Here's how the part is built. I have some questions about the finished solid (model axes, mm). Coordinates: 2 decimals unless noted, no trailing zeros. Order: outer loops, then holes, each group sorted by start corner. A loop starts at its lowest first (then second) coordinate and runs counter-clockwise, first axis right, second up. Notation, with made-up numbers: (-29, -17) - (26, -17) arc R17 ccw to (26, 1) - close; hole circle Ø1 at (75, -1). An arc over 180 degrees is marked (long way). Answer as CSV lines item,"result". Start each with the question number.
Item 1: Imagine slicing it at A-A on y = 30.5. List the corners of the cut face in (x, z) for me (3 decimals).
Item 2: Imagine slicing it at B-B on z = 250. List the corners of the cut face in (x, y) for me (3 decimals).
Item 3: I'm going to push flat-ended pins straight in: pin 1 (2.5 mm diameter, centred on x = 0, z = 241.3, fed in from +Y) (3 decimals); pin 2 (5 mm diameter, centred on x = 0, z = 139.7, fed in from +Y); pin 3 (12 mm diameter, centred on x = -2.5, y = -26, fed in from +Z). Where does each tip first touch, or does it pass through?
Item 4: I need wall thicknesses on line 1 (Y direction, x = 3.25, z = 158) (3 decimals); line 2 (X direction, y = 37.3, z = 165.1); line 3 (X direction, y = -7, z = 205) (3 decimals). Which ranges of each line are inside material? Lowest first, please.
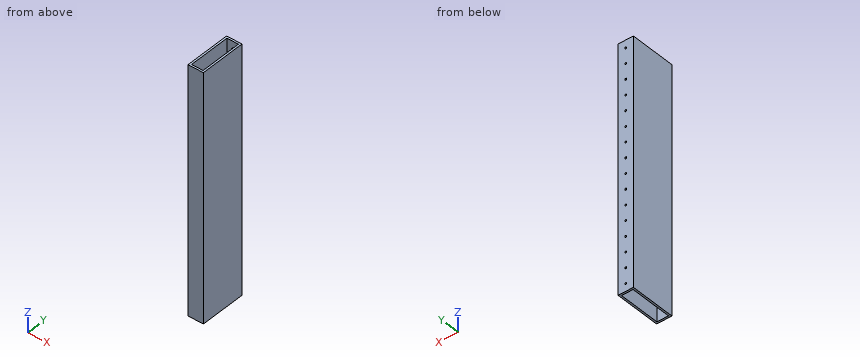
from build123d import *

# Parameters (mm, degrees)
SKETCH1_W           = 25.4
SKETCH1_H           = 76.2
BOSS_EXTRUDE1_DEPTH = 406.4
SHELL1_T            = -3.175
SKETCH2_R           = 1.5875
CUT_EXTRUDE1_DEPTH  = 3.175
LPATTERN1_COUNT     = 16
LPATTERN1_PITCH     = 25.4


with BuildPart() as part:
    # Sketch1 → Boss-Extrude1 (new body)
    with BuildSketch(Plane.XY):
        Rectangle(SKETCH1_W, SKETCH1_H)
    extrude(amount=BOSS_EXTRUDE1_DEPTH)

    # Shell1
    shell1_openings = [part.faces().sort_by_distance(p)[0] for p in [
        (0, 0, 406.4),
        (0, 0, 0),
    ]]
    offset(amount=SHELL1_T, openings=shell1_openings, kind=Kind.INTERSECTION)

    # Sketch2 → Cut-Extrude1 (cut)
    with BuildSketch(Plane(origin=(0, 38.1, 0), x_dir=(1, 0, 0), z_dir=(0, 1, 0))):
        with Locations((0, -12.7)):
            Circle(SKETCH2_R)
    cut_extrude1 = extrude(amount=-CUT_EXTRUDE1_DEPTH, mode=Mode.SUBTRACT)

    # LPattern1: Cut-Extrude1 ×16
    with Locations(*[(0, 0, i * LPATTERN1_PITCH) for i in range(1, LPATTERN1_COUNT)]):
        add(cut_extrude1, mode=Mode.SUBTRACT)


solid = part.part
Responses:
1,outline,"(-12.7, 0) - (-9.525, 0) - (-9.525, 406.4) - (-12.7, 406.4) - close; (9.525, 0) - (12.7, 0) - (12.7, 406.4) - (9.525, 406.4) - close"
2,outline,"(-12.7, -38.1) - (12.7, -38.1) - (12.7, 38.1) - (-12.7, 38.1) - close; hole (-9.525, -34.925) - (9.525, -34.925) - (9.525, 34.925) - (-9.525, 34.925) - close"
3,pin 1,"stops at y = -34.925"
3,pin 2,"stops at y = 38.1"
3,pin 3,"passes through"
4,line 1,"y = -38.1 to -34.925, 34.925 to 38.1"
4,line 2,"x = -12.7 to -1.59, 1.59 to 12.7"
4,line 3,"x = -12.7 to -9.525, 9.525 to 12.7"
